Print and shaded views of the part. All mm, measured from the part's lowest x, y and z. Coordinates: 2 decimals unless noted, no trailing zeros. Loops run counter-clockwise (first coordinate to the right, second up) from the corner with the lowest first, then second, coordinate; pieces in that order, holes last.
1) Wall check: line 1 along Z through (x, y) = (3, 1.6); line 2 along Z through (x, y) = (1.95, 0.25); line 3 along X through (y, z) = (0.4, 49.5). Give the ranges that are in metal, low to high.
2) Saw through at B-B, the plane x = 3. Write the cut outline in (y, z), and give its area (3 significant figures).
3) Saw through at C-C, the plane y = 1.7. Write the cut outline in (x, z).
4) Pin check, flat tip, straight feed: pin 1 Ø1 at (x, y) = (0.5, 1) entering from -Z. Stop position of the tip, or through.
5) Saw through at A-A, the plane z = 49. Write the cut outline in (x, y).
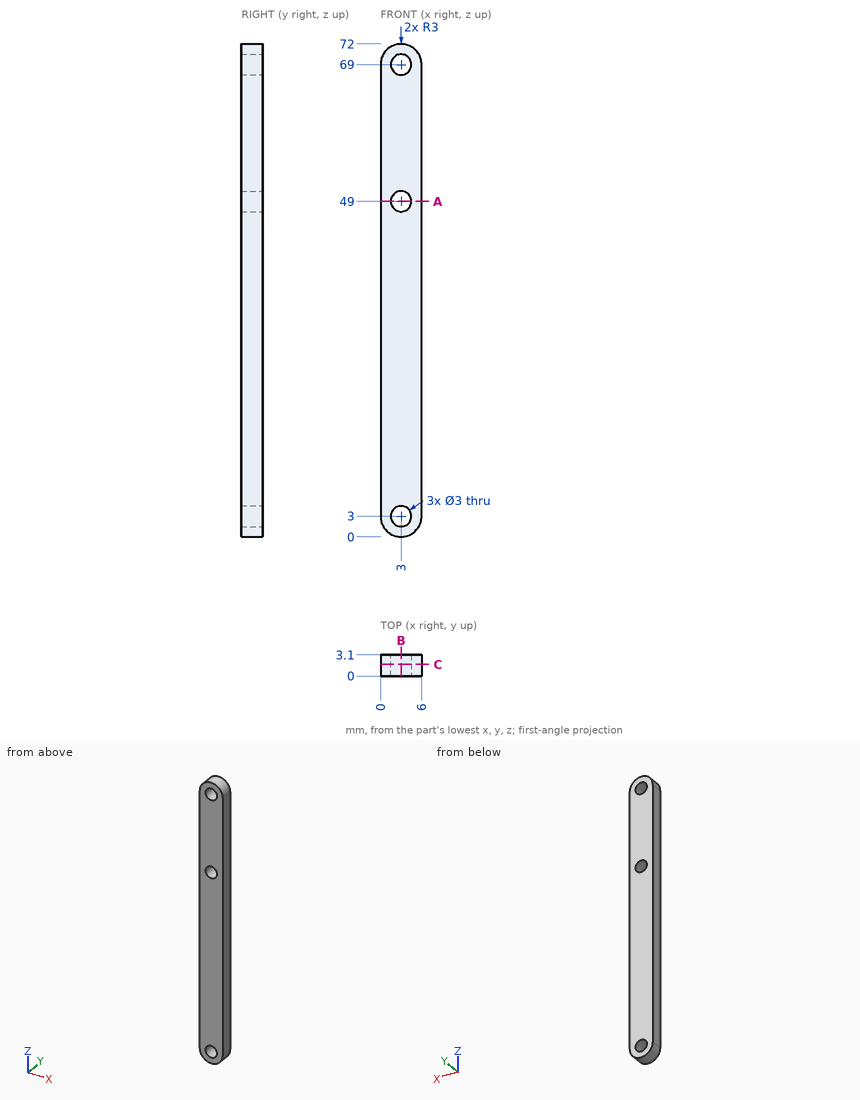
Data:
1. line 1: z = 0 to 1.5, 4.5 to 47.5, 50.5 to 67.5, 70.5 to 72
1. line 2: z = 0.19 to 1.93, 4.07 to 47.93, 50.07 to 67.93, 70.07 to 71.81
1. line 3: x = 0 to 1.59, 4.41 to 6
2. outline: (0, 0) - (3.1, 0) - (3.1, 1.5) - (0, 1.5) - close; (0, 4.5) - (3.1, 4.5) - (3.1, 47.5) - (0, 47.5) - close; (0, 50.5) - (3.1, 50.5) - (3.1, 67.5) - (0, 67.5) - close; (0, 70.5) - (3.1, 70.5) - (3.1, 72) - (0, 72) - close
2. area: 195 mm2
3. outline: (0, 3) arc R3 ccw to (6, 3) - (6, 69) arc R3 ccw to (0, 69) - close; hole circle Ø3 at (3, 3); hole circle Ø3 at (3, 49); hole circle Ø3 at (3, 69)
4. pin 1: stops at z = 0.76
5. outline: (0, 0) - (1.5, 0) - (1.5, 3.1) - (0, 3.1) - close; (4.5, 0) - (6, 0) - (6, 3.1) - (4.5, 3.1) - close
